Check sheet for the modelled part. Datum: model origin and axes. Units: mm. A direction names the side the tool comes from. Give positions to 0.01 mm unless a question says otherwise; leave off trailing zeros. Write each loop counter-clockwise with the first axis right and the second up, starting at its lowest first coordinate (ties: lowest second). Pieces come first, ordered by that corner, then holes. Notation, with made-up numbers: (25.5, 55) -> (65.5, 55) arc R29 cw to (65.5, 77) -> close; hole circle Ø10 at (51, 37). An arc over 180 degrees is marked (long way). Return JSON: item names as keys, results as strings.
from build123d import *

# Parameters (mm, degrees)
F0_W          = 35.36984
F0_H          = 86.427912
F1_DEPTH      = 25.4
F1_DEPTH_BACK = 26.416
F2_T          = -2.54


with BuildPart() as f1:
    # F0 (on Top) → F1 (new body, two sides)
    with BuildSketch(Plane.XY) as f1_sk:
        Polygon((-9.412942, 58.046471), (-17.68492, 43.213956), (17.68492, 43.213956), (9.698181, 58.046471), align=None)
        Rectangle(F0_W, F0_H)
    extrude(amount=F1_DEPTH)
    extrude(f1_sk.sketch, amount=-F1_DEPTH_BACK)

    # F2
    f2_openings = [f1.faces().sort_by_distance(p)[0] for p in [
        (-13.548931, 50.630214, -0.508),
        (13.691551, 50.630214, -0.508),
    ]]
    offset(amount=F2_T, openings=f2_openings)


solid = f1.part
(1) Cross-section at B-B on z = 17. Enter the section's corners in (x, y).
Reply:
{"outline": "(-17.68, -43.21) -> (17.68, -43.21) -> (17.68, 43.21) -> (15.14, 47.93) -> (15.14, -40.67) -> (-15.14, -40.67) -> (-15.14, 47.77) -> (-17.68, 43.21) -> close; (-10.83, 55.51) -> (11.07, 55.51) -> (9.7, 58.05) -> (-9.41, 58.05) -> close"}
(2) Set-up check for faces 4 (the flat face through (-15.145, 3, 0)), 5 (the flat face through (0, 8, -26.416)), 6 (the flat face through (0, 8, -23.876)), 7 (the flat face through (0, 55.506, 0)): record each of +Z, -Z, +X, -X, +Y, -Y from which the full face is reachable in a straight line by a thin tool's end or side.
Reply:
{"face 4": "+Y", "face 5": "-Z, +X, -X, +Y, -Y", "face 6": "none", "face 7": "+X, -X"}
(3) Depth check by flat-ended pin: pin 1 Ø3 at (y, z) = (47, -4.5) entering from +X. Enter the tip coordinate at first touch or a pass-through.
Reply:
{"pin 1": "x = 16.45"}
(4) Cross-section at A-A on x = -1. Enter the section's corners in (y, z).
Reply:
{"outline": "(-43.21, -26.42) -> (58.05, -26.42) -> (58.05, 25.4) -> (-43.21, 25.4) -> close; hole (-40.67, -23.88) -> (55.51, -23.88) -> (55.51, 22.86) -> (-40.67, 22.86) -> close"}
(5) Release check for a two-part mould opening along X. For faces 1 (the flat face through (15.145, 3, 0)), 2 (the flat face through (0, 58.046, 0)), 3 (the flat face through (-15.33, 47.44, -0.15)) record: pulls with the +X half, pulls with the -X half, needs draft (parallel to the pull), parting line crosses it, or undercut.
Reply:
{"face 1": "undercut", "face 2": "needs draft", "face 3": "pulls with the -X half"}
(6) Cross-section at D-D on y = 51. Enter the section's corners in (x, z).
Reply:
{"outline": "(-13.34, -26.42) -> (13.49, -26.42) -> (13.49, -23.88) -> (-13.34, -23.88) -> close; (-13.34, 22.86) -> (13.49, 22.86) -> (13.49, 25.4) -> (-13.34, 25.4) -> close"}
(7) Cross-section at C-C on y = -12.5. Enter the section's corners in (x, z).
Reply:
{"outline": "(-17.68, -26.42) -> (17.68, -26.42) -> (17.68, 25.4) -> (-17.68, 25.4) -> close; hole (-15.14, -23.88) -> (15.14, -23.88) -> (15.14, 22.86) -> (-15.14, 22.86) -> close"}
(8) Thickness scan on L1, parallel to Y at x = 7.5, z = 16; L2, parallel to Z at x = -5, y = -20.5; L3, parallel to X at y = -17, z = 4. Record the ranges inside material, lowest first.
Reply:
{"L1": "-43.21 to -40.67, 55.51 to 58.05", "L2": "-26.42 to -23.88, 22.86 to 25.4", "L3": "-17.68 to -15.14, 15.14 to 17.68"}
